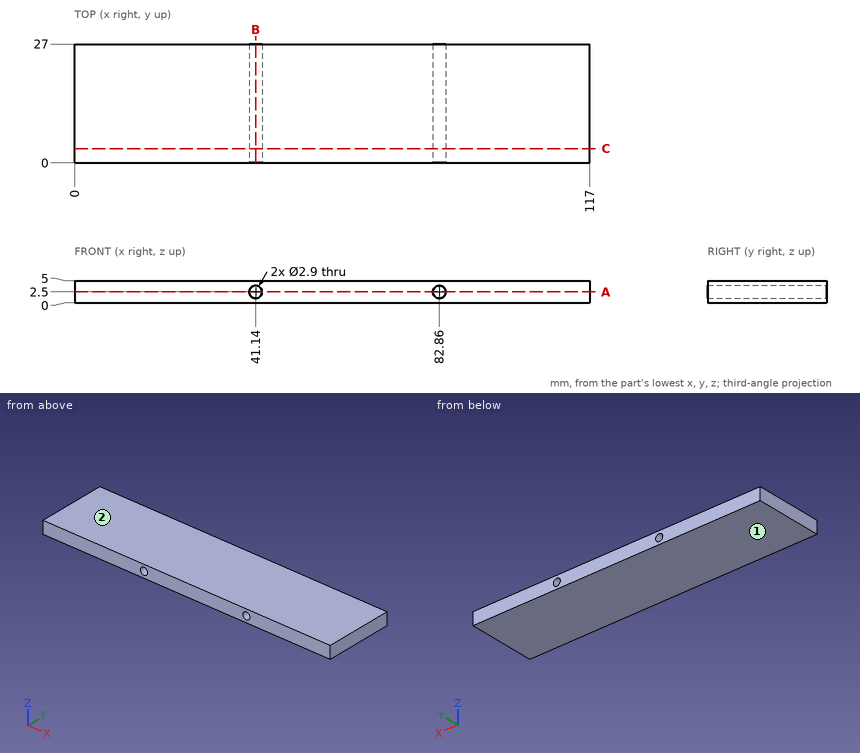
Study the drawing (mm; zero at the part's minimum x, y, z) and answer. Give positions to 0.01 mm unless a question says otherwise; leave off trailing zeros. Loops run counter-clockwise (first coordinate to the right, second up) from the corner with the lowest first, then second, coordinate; pieces in that order, holes last. Notation, with made-up numbers: (22.5, 2) -> (75.5, 2) arc R22 ccw to (75.5, 25) -> close; hole circle Ø10 at (44.5, 75.5). An arc over 180 degrees is marked (long way). Use a Markdown table: item, result. Add a question column.
1) For a pull along Z with two mould halves and no side action, classify the marked faces 1 and 2 as +Z half, -Z half, draft (parallel to the pull), parting line (faces both ways), or undercut.
2) The part is cut by section A-A, the plane z = 2.5. Determine the outline of the cut face in (x, y).
3) The part is cut by section C-C, the plane y = 3.25. Determine the outline of the cut face in (x, z).
4) The part is cut by section B-B, the plane x = 41.14. Determine the outline of the cut face in (y, z), plus the area to 3 significant figures.
5) Consider line 1 along X through (y, z) = (15.25, 2.5); line 2 along Z through (x, y) = (82.86, 19.5); line 3 along X through (y, z) = (14.5, 3.1). Determine where each line is inside the solid, lowest interval first.
6) This flat-tipped pin is pushed along its axis until it touches: P1, Ø10, axis at x = 13, y = 24, coming from the -Z side. Where does it stop, or does it pass through?
Reported:
| question | item | result |
|---|---|---|
| 1 | face 1 | -Z half |
| 1 | face 2 | +Z half |
| 2 | outline | (0, 0) -> (39.69, 0) -> (39.69, 27) -> (0, 27) -> close; (42.59, 0) -> (81.41, 0) -> (81.41, 27) -> (42.59, 27) -> close; (84.31, 0) -> (117, 0) -> (117, 27) -> (84.31, 27) -> close |
| 3 | outline | (0, 0) -> (117, 0) -> (117, 5) -> (0, 5) -> close; hole circle Ø2.9 at (41.14, 2.5); hole circle Ø2.9 at (82.86, 2.5) |
| 4 | outline | (0, 0) -> (27, 0) -> (27, 1.05) -> (0, 1.05) -> close; (0, 3.95) -> (27, 3.95) -> (27, 5) -> (0, 5) -> close |
| 4 | area | 56.7 mm^2 |
| 5 | line 1 | x = 0 to 39.69, 42.59 to 81.41, 84.31 to 117 |
| 5 | line 2 | z = 0 to 1.05, 3.95 to 5 |
| 5 | line 3 | x = 0 to 39.82, 42.46 to 81.54, 84.18 to 117 |
| 6 | P1 | stops at z = 0 |
